from build123d import *

# Parameters (mm, degrees)
F1_DEPTH = 12.7
F3_DEPTH = 25.4
F4_W     = 13.24638
F4_H     = 9.920692
F5_DEPTH = 15.927161


with BuildPart() as f1:
    # F0 (on Top) → F1 (new body)
    with BuildSketch(Plane.XY):
        with BuildLine():
            Line((-53.466398, -11.755024), (56.120757, -11.755024))
            Line((56.120757, -11.755024), (56.120757, -6.333794))
            ThreePointArc((56.120757, -6.333794), (46.333815, 0), (56.120757, 6.333794))
            Line((56.120757, 6.333794), (56.120757, 11.755024))
            Line((56.120757, 11.755024), (-53.466398, 11.755024))
            Line((-53.466398, 11.755024), (-53.466398, 5.315492))
            ThreePointArc((-53.466398, 5.315492), (-48.620146, 4.412441), (-46.421961, 0))
            ThreePointArc((-46.421961, 0), (-48.620146, -4.412441), (-53.466398, -5.315492))
            Line((-53.466398, -5.315492), (-53.466398, -11.755024))
        make_face()
        with BuildLine():
            Line((56.120757, -6.333794), (56.120757, -11.755024))
            ThreePointArc((56.120757, -11.755024), (67.875781, 0), (56.120757, 11.755024))
            Line((56.120757, 11.755024), (56.120757, 6.333794))
            ThreePointArc((56.120757, 6.333794), (59.105633, 3.772233), (60.219784, 0))
            ThreePointArc((60.219784, 0), (59.105633, -3.772233), (56.120757, -6.333794))
        make_face()
        with BuildLine():
            ThreePointArc((-53.466398, 11.755024), (-65.221422, 0), (-53.466398, -11.755024))
            Line((-53.466398, -11.755024), (-53.466398, -5.315492))
            ThreePointArc((-53.466398, -5.315492), (-57.477287, 0), (-53.466398, 5.315492))
            Line((-53.466398, 5.315492), (-53.466398, 11.755024))
        make_face()
    extrude(amount=F1_DEPTH)

    # F2 (on Right) → F3 (join)
    with BuildSketch(Plane.YZ):
        with BuildLine():
            Line((-4.171137, 29.520769), (-4.171137, 11.186233))
            Line((-4.171137, 11.186233), (4.171137, 11.186233))
            Line((4.171137, 11.186233), (4.171137, 29.520769))
            ThreePointArc((4.171137, 29.520769), (0, 25.349631), (-4.171137, 29.520769))
        make_face()
        with BuildLine():
            ThreePointArc((4.171137, 29.520769), (0, 33.691906), (-4.171137, 29.520769))
            Line((-4.171137, 29.520769), (-2.292054, 29.520769))
            ThreePointArc((-2.292054, 29.520769), (0, 31.812823), (2.292054, 29.520769))
            Line((2.292054, 29.520769), (4.171137, 29.520769))
        make_face()
        with BuildLine():
            Line((-2.292054, 29.520769), (-4.171137, 29.520769))
            ThreePointArc((-4.171137, 29.520769), (0, 25.349631), (4.171137, 29.520769))
            Line((4.171137, 29.520769), (2.292054, 29.520769))
            ThreePointArc((2.292054, 29.520769), (0, 27.228715), (-2.292054, 29.520769))
        make_face()
    extrude(amount=F3_DEPTH)

    # F4 (on face) → F5 (cut, through all)
    with BuildSketch(Plane.XZ.offset(4.171137)):
        with Locations((13.116183, 28.764711)):
            Rectangle(F4_W, F4_H)
        with BuildLine():
            Line((19.739373, 23.804365), (6.492993, 23.804365))
            ThreePointArc((6.492993, 23.804365), (13.116183, 17.181175), (19.739373, 23.804365))
        make_face()
    extrude(amount=-F5_DEPTH, mode=Mode.SUBTRACT)


solid = f1.part
The model under review builds one solid part; all positions refer to its coordinate system, in mm. A direction names the side the tool comes from. Give positions to 0.01 mm unless a question says otherwise; leave off trailing zeros. Loops run counter-clockwise (first coordinate to the right, second up) from the corner with the lowest first, then second, coordinate; pieces in that order, holes last. Notation, with made-up numbers: (62, 66.25) -> (99, 66.25) arc R21 ccw to (99, 101.25) -> close; hole circle Ø8 at (79, 6.25). An arc over 180 degrees is marked (long way). Answer as a JSON object with one key per item and string values. Group by question number.
Q1. Take a section at C-C (x = 21). Write out the cut boundary in (y, z).
Q2. Tool access review of faces 1 (the flat face through (25.4, 0, 23)), 2 (the flat face through (6.493, 0, 26)), 3 (the flat face through (1, -11.755, 6)), 4 (the flat face through (10, -4.171, 17)): name each direction out of +Z, -Z, +X, -X, +Y, -Y from which nothing blocks a thin tool from reaching the whole face with its end or side.
Q3. Insertion check: pin 1 (2.5 mm diameter, centred on y = 1.5, z = 31, fed in from +X); pin 2 (3 mm diameter, centred on y = 0, z = 29.52, fed in from -X); pin 3 (13.5 mm diameter, centred on x = 7, z = 20, fed in from +Y); pin 4 (1 mm diameter, centred on x = 28.5, y = 9, fed in from -Z). Each pin has a flat end and moves straight along its axis. Give the tip position at first contact, or say it passes through.
Q4. Take a section at D-D (x = -29). Write out the cut boundary in (y, z), plus the area to 3 significant figures.
Q5. Take a section at B-B (z = 8). Write out the cut boundary in (x, y), plus the area to 3 significant figures.
Q6. Wall thickness on line 1 along X through (y, z) = (0, 2.75); line 2 along Z through (x, y) = (1.75, 0); line 3 along Z through (x, y) = (-42.5, -7): over which ranges is each line inside the solid? List them lowest first.
Q7. Take a section at A-A (z = 25). Write out the cut boundary in (x, y).
Q8. Draft analysis for pull direction X (two halves, no side actions). For faces 5 (the flat face through (19.739, 0, 26)), 6 (the flat face through (0, 0, 23)), 7 (the flat face through (10, 4.171, 17)), state which applies: pulls with the +X half, pulls with the -X half, needs draft (parallel to the pull), parting line crosses it, or undercut.
Answer below:
{
 "1": {"outline": "(-11.76, 0) -> (11.76, 0) -> (11.76, 12.7) -> (4.17, 12.7) -> (4.17, 29.52) arc R4.17 ccw to (-4.17, 29.52) -> (-4.17, 12.7) -> (-11.76, 12.7) -> close; hole circle Ø4.58 at (0, 29.52)"},
 "2": {"face 1": "+Z, +X, +Y, -Y", "face 2": "+Z, +Y, -Y", "face 3": "+Z, -Z, +X, -X, -Y", "face 4": "+Z, +X, -X, -Y"},
 "3": {"pin 1": "stops at x = 25.4", "pin 2": "passes through", "pin 3": "stops at y = 4.17", "pin 4": "stops at z = 0"},
 "4": {"outline": "(-11.76, 0) -> (11.76, 0) -> (11.76, 12.7) -> (-11.76, 12.7) -> close", "area": "299 mm2"},
 "5": {"outline": "(-53.47, -11.76) -> (56.12, -11.76) arc R11.76 ccw to (56.12, 11.76) -> (-53.47, 11.76) arc R11.76 ccw to start; hole circle Ø11.06 at (-51.95, 0); hole (56.12, -6.33) arc R6.94 ccw to (60.22, 0) arc R6.94 ccw to (56.12, 6.33) arc R6.94 ccw (long way) to start", "area": "2,760 mm2"},
 "6": {"line 1": "x = -65.22 to -57.48, -46.42 to 46.33, 60.22 to 67.88", "line 2": "z = 0 to 27.23, 31.81 to 33.69", "line 3": "z = 0 to 12.7"},
 "7": {"outline": "(0, -4.17) -> (6.49, -4.17) -> (6.49, 4.17) -> (0, 4.17) -> close; (19.74, -4.17) -> (25.4, -4.17) -> (25.4, 4.17) -> (19.74, 4.17) -> close"},
 "8": {"face 5": "undercut", "face 6": "pulls with the -X half", "face 7": "needs draft"}
}
